Source: CAD feature listing. Evaluate the final solid. Frame: model axes, mm. A direction names the side the tool comes from. Give positions to 0.01 mm unless a question says otherwise; leave off trailing zeros. Write each loop counter-clockwise with the first axis right and the second up, starting at its lowest first coordinate (ties: lowest second). Pieces come first, ordered by that corner, then holes.
Autodesk Inventor part; units mm, degrees
ref_plane "YZ Plane" through (0, 0, 0) normal (1, 0, 0) x (0, 1, 0)
ref_plane "XZ Plane" through (0, 0, 0) normal (0, 1, 0) x (-1, 0, 0)
ref_plane "XY Plane" through (0, 0, 0) normal (0, 0, 1) x (1, 0, 0)
sketch "Sketch1" plane through (0, 0, 0) normal (0, 1, 0) x (-1, 0, 0)
  circle A0 centre (0, 0) radius 10
  dimension "d0" = 20
extrude "Extrusion1" add sketch "Sketch1" along normal blind 15
fillet "Fillet1" radius 2.5 1 edges at (10, 15, 0)
sketch "Sketch2" plane through (0, 15, 0) normal (0, 1, 0) x (1, 0, 0)
  line L0 (-4.9845, 3.1153) -> (3.7384, 3.1153) construction
  line L1 (3.7384, 3.1153) -> (3.7384, -3.4029) construction
  line L2 (3.7384, -3.4029) -> (-4.9845, -3.4029) construction
  line L3 (-4.9845, -3.4029) -> (-4.9845, 3.1153) construction
  spline S0 degree 2 poles (-2.236, -3.1132) (-2.7748, -3.1132) (-3.5756, -2.8315) (-3.8574, -2.5497) knots 0 0 0 1 2 2 2
  spline S1 degree 2 poles (-3.8574, -2.5497) (-4.1787, -2.2333) (-4.4407, -1.3435) (-4.4407, -0.691) knots 0 0 0 1 2 2 2
  line L4 (-4.4407, -0.691) -> (-4.4407, 3.1153)
  line L5 (-4.4407, 3.1153) -> (-3.63, 3.1153)
  line L6 (-3.63, 3.1153) -> (-3.63, -0.691)
  spline S2 degree 2 poles (-3.63, -0.691) (-3.63, -1.1162) (-3.5213, -1.6896) (-3.368, -1.9219) knots 0 0 0 1 2 2 2
  spline S3 degree 2 poles (-3.368, -1.9219) (-3.2049, -2.1691) (-2.6414, -2.4212) (-2.236, -2.4212) knots 0 0 0 1 2 2 2
  spline S4 degree 2 poles (-2.236, -2.4212) (-1.8554, -2.4212) (-1.2622, -2.1691) (-1.0991, -1.9219) knots 0 0 0 1 2 2 2
  spline S5 degree 2 poles (-1.0991, -1.9219) (-0.9458, -1.6896) (-0.8371, -1.1211) (-0.8371, -0.7108) knots 0 0 0 1 2 2 2
  line L7 (-0.8371, -0.7108) -> (-0.8371, 3.1153)
  line L8 (-0.8371, 3.1153) -> (-0.0264, 3.1153)
  line L9 (-0.0264, 3.1153) -> (-0.0264, -0.691)
  spline S6 degree 2 poles (-0.0264, -0.691) (-0.0264, -1.3287) (-0.2834, -2.2383) (-0.6097, -2.5497) knots 0 0 0 1 2 2 2
  spline S7 degree 2 poles (-0.6097, -2.5497) (-0.9013, -2.8364) (-1.6725, -3.1132) (-2.236, -3.1132) knots 0 0 0 1 2 2 2
  spline S8 degree 2 poles (4.9911, 1.2764) (4.9911, 0.8809) (4.7093, 0.1691) (4.4572, -0.0781) knots 0 0 0 1 2 2 2
  spline S9 degree 2 poles (4.4572, -0.0781) (4.1408, -0.3895) (3.2856, -0.7108) (2.6331, -0.7108) knots 0 0 0 1 2 2 2
  line L10 (2.6331, -0.7108) -> (1.946, -0.7108)
  line L11 (1.946, -0.7108) -> (1.946, -2.9847)
  line L12 (1.946, -2.9847) -> (1.1353, -2.9847)
  line L13 (1.1353, -2.9847) -> (1.1353, 3.1153)
  line L14 (1.1353, 3.1153) -> (2.6677, 3.1153)
  spline S10 degree 2 poles (2.6677, 3.1153) (3.2115, 3.1153) (3.9727, 2.9373) (4.2644, 2.7347) knots 0 0 0 1 2 2 2
  spline S11 degree 2 poles (4.2644, 2.7347) (4.6055, 2.5023) (4.9911, 1.7856) (4.9911, 1.2764) knots 0 0 0 1 2 2 2
  spline S12 degree 2 poles (4.1458, 1.2517) (4.1458, 1.568) (3.9283, 2.0327) (3.7058, 2.181) knots 0 0 0 1 2 2 2
  spline S13 degree 2 poles (3.7058, 2.181) (3.513, 2.3095) (2.9989, 2.4133) (2.6183, 2.4133) knots 0 0 0 1 2 2 2
  line L15 (2.6183, 2.4133) -> (1.946, 2.4133)
  line L16 (1.946, 2.4133) -> (1.946, -0.0187)
  line L17 (1.946, -0.0187) -> (2.4996, -0.0187)
  spline S14 degree 2 poles (2.4996, -0.0187) (2.994, -0.0187) (3.602, 0.1394) (3.7997, 0.3471) knots 0 0 0 1 2 2 2
  spline S15 degree 2 poles (3.7997, 0.3471) (3.9826, 0.53) (4.1458, 0.96) (4.1458, 1.2517) knots 0 0 0 1 2 2 2
  point P0 (0, 0)
extrude "Extrusion2" cut sketch "Sketch2" against normal blind 5
sketch "Sketch3" plane through (0, 0, 0) normal (0, -1, 0) x (1, 0, 0)
  circle A0 centre (0, 0) radius 7.5
extrude "Extrusion3" cut sketch "Sketch3" against normal blind 2.5
properties part number "UP Button"
1. Access query for faces 1 (the flat face through (-4, 0, 7)), 2 (the flat face through (-4, 10, 0)), 3 (the cylindrical face through (-7.493, 1.232, 0.33)). Directions: +Z, -Z, +X, -X, +Y, -Y. A direction counts if a zero-diameter tool reaches every point of the face in a straight line with its end or side. Return the directions, or none.
2. Cut plane A-A, the plane y = 10.75. State how many separate pieces and enclosed holes the cut face has, then the cut area to 3 significant figures.
3. Mould query, pull axis X, two halves, no side actions, for faces 4 (the flat face through (0, 2.5, 0)), 5 (the cylindrical face through (2.17, 6.16, 9.76)), 6 (the flat face through (3, 15, -1)), 7 (the flat face through (1.75, 10, -0.79)). Classes: +X half, -X half, draft (parallel to the pull), parting line (faces both ways), or undercut.
4. Contact query for flat-ended pins moving along their axis: P1, Ø1.7, axis at x = 1.5, y = 11.5, coming from the +Z side; P2, Ø3, axis at y = 8.5, z = 0.5, coming from the -X side; P3, Ø3, axis at x = 6, y = 11.5, coming from the -Z side; P4, Ø0.7, axis at x = 2, y = 12.5, coming from the -Z side. Output: stop coordinate, or through.
5. Cut plane B-B, the plane y = 8.75. Return the cut outline in (x, z).
6. Line query: L1, parallel to Z at x = 0, y = 0.75; L2, parallel to Y at x = -4.5, z = -5.25; L3, parallel to Z at x = -1, y = 2.25. Output: solid intervals per line, ascending.
Response values:
1. face 1: +Z, -Z, +X, -X, -Y
1. face 2: +Y
1. face 3: -Y
2. separate pieces: 2
2. enclosed holes: 2
2. area: 293 mm2
3. face 4: undercut
3. face 5: parting line
3. face 6: draft
3. face 7: undercut
4. P1: stops at z = 9.98
4. P2: stops at x = -10
4. P3: stops at z = -8.93
4. P4: stops at z = -9.86
5. outline: circle Ø20 at (0, 0)
6. L1: z = -10 to -7.5, 7.5 to 10
6. L2: y = 2.5 to 15
6. L3: z = -9.95 to -7.43, 7.43 to 9.95
